Input: dimensioned drawing with shaded views. Units: mm. Origin: part minimum x, y, z. Give positions to 0.01 mm unless a question says otherwise; leave off trailing zeros. Write each loop counter-clockwise with the first axis right and the second up, starting at its lowest first coordinate (ties: lowest second). Pieces come first, ordered by that corner, then holes.
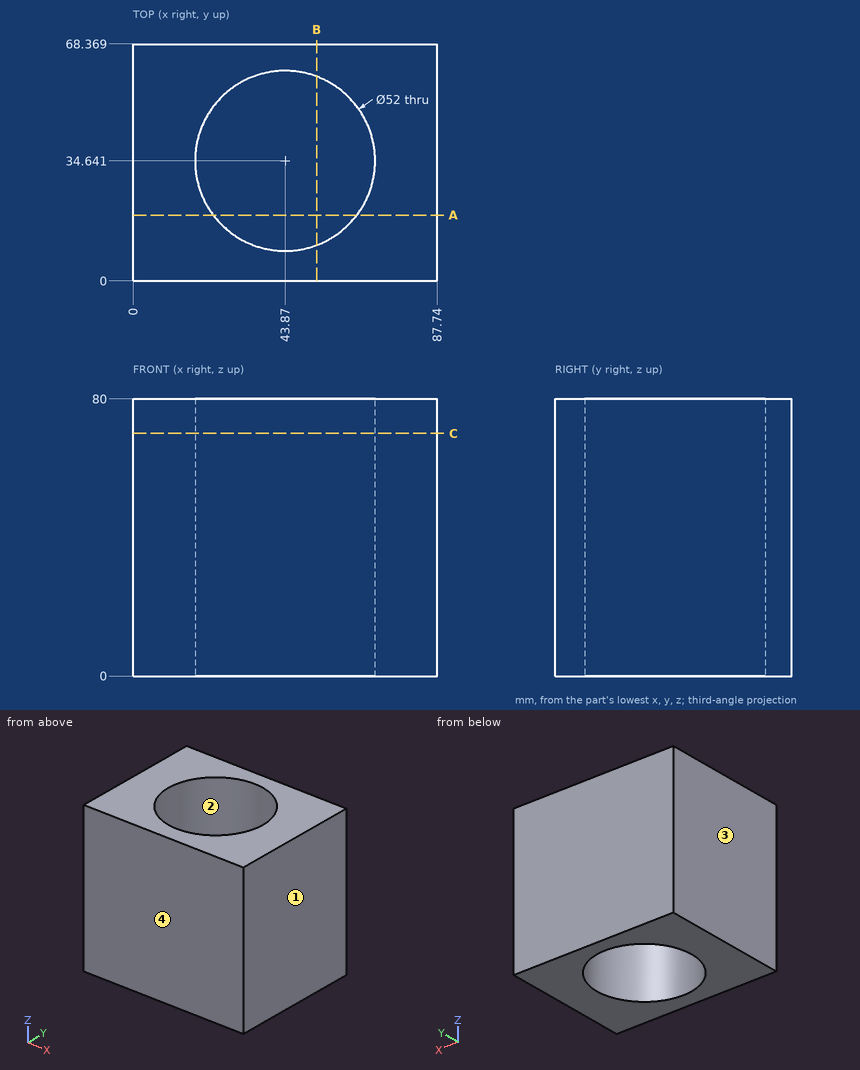
Item 1: Line query: L1, parallel to Y at x = 44.5, z = 73; L2, parallel to X at y = 23.5, z = 37; L3, parallel to X at y = 35.5, z = 10 (1 decimal). Output: solid intervals per line, ascending.
Found:
L1: y = 0 to 8.65, 60.63 to 68.37
L2: x = 0 to 20.38, 67.36 to 87.74
L3: x = 0 to 17.9, 69.9 to 87.7
Item 2: Section B-B, the plane x = 53. Return the cut outline in (y, z) (1 decimal), plus the area to 3 significant figures.
Found:
outline: (0, 0) - (10.3, 0) - (10.3, 80) - (0, 80) - close; (59, 0) - (68.4, 0) - (68.4, 80) - (59, 80) - close
area: 1,570 mm2
Item 3: Section C-C, the plane z = 70. Return the cut outline in (x, y).
Found:
outline: (0, 0) - (87.74, 0) - (87.74, 68.37) - (0, 68.37) - close; hole circle Ø52 at (43.87, 34.64)
Item 4: Pin query (flat end, axial travel): pin 1 Ø3 at (y, z) = (31.5, 59) entering from -X. Return the tip coordinate at first contact, or that it passes through.
Found:
pin 1: stops at x = 0
Item 5: Section A-A, the plane y = 19. Return the cut outline in (x, z).
Found:
outline: (0, 0) - (23.1, 0) - (23.1, 80) - (0, 80) - close; (64.64, 0) - (87.74, 0) - (87.74, 80) - (64.64, 80) - close
Item 6: Pull-direction query (X, two-part tool) for the marked faces 1, 2, 3 and 4; classes: +X half, -X half, draft (parallel to the pull), parting line (faces both ways), or undercut.
Found:
face 1: +X half
face 2: undercut
face 3: -X half
face 4: draft
